Part print with two shaded views. Sizes in mm from the minimum x, y, z corner. Round coordinates to 2 decimals unless told otherwise and drop trailing zeros. Loops run counter-clockwise (first coordinate to the right, second up) from the corner with the lowest first, then second, coordinate; pieces in that order, holes last.
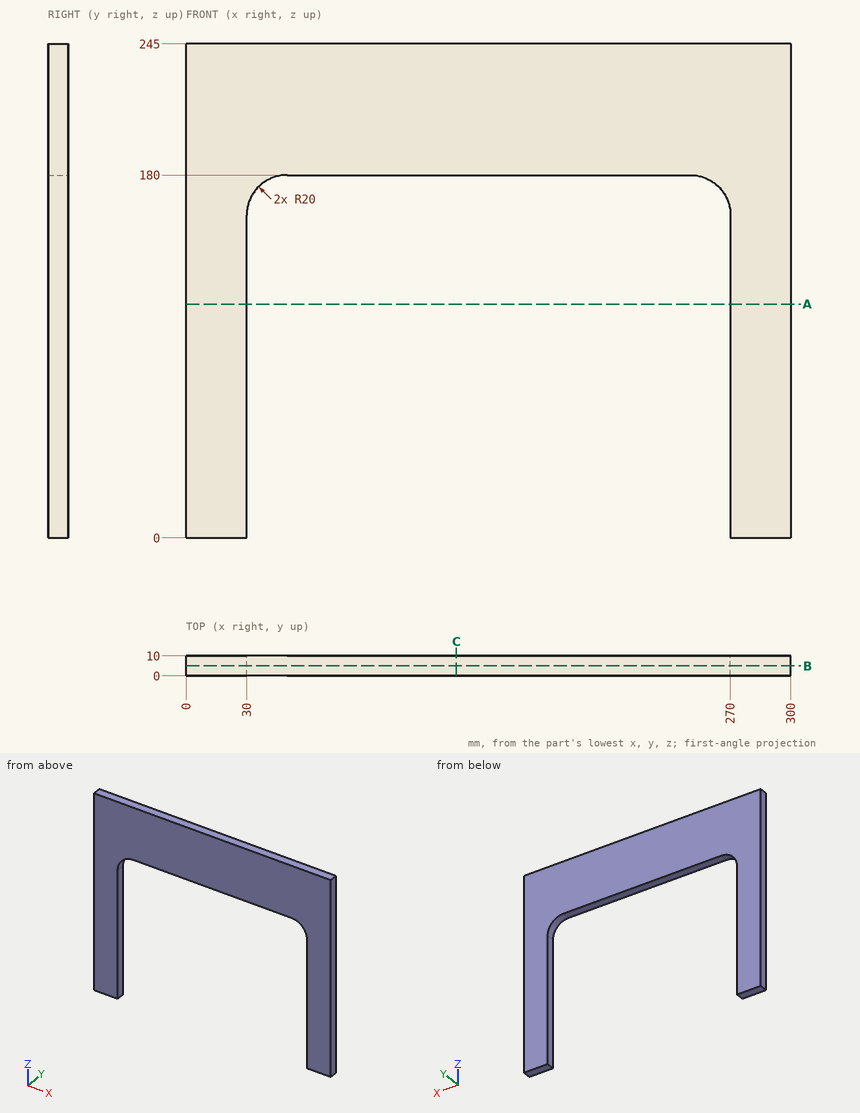
Item 1: Cut at B-B (y = 5). List the corners of the cut face in (x, z).
Verdict:
outline: (0, 0) - (30, 0) - (30, 160) arc R20 cw to (50, 180) - (250, 180) arc R20 cw to (270, 160) - (270, 0) - (300, 0) - (300, 245) - (0, 245) - close
Item 2: Cut at C-C (x = 134). List the corners of the cut face in (y, z), plus the area to 3 significant figures.
Verdict:
outline: (0, 180) - (10, 180) - (10, 245) - (0, 245) - close
area: 650 mm2
Item 3: Wall check: L1, parallel to X at y = 7.5, z = 57; L2, parallel to Z at x = 81.5, y = 7.5; L3, parallel to Z at x = 251.5, y = 7.25. Give the ranges that are in metal, low to high.
Verdict:
L1: x = 0 to 30, 270 to 300
L2: z = 180 to 245
L3: z = 179.94 to 245
Item 4: Flat gauge pins, fed straight in: P1, Ø4, axis at y = 5.5, z = 192, coming from the -X side; P2, Ø4, axis at x = 210, y = 6, coming from the -Z side. Where does each tip first touch, or does it go through?
Verdict:
P1: stops at x = 0
P2: stops at z = 180
Item 5: Cut at A-A (z = 116). List the corners of the cut face in (x, y).
Verdict:
outline: (0, 0) - (30, 0) - (30, 10) - (0, 10) - close; (270, 0) - (300, 0) - (300, 10) - (270, 10) - close
